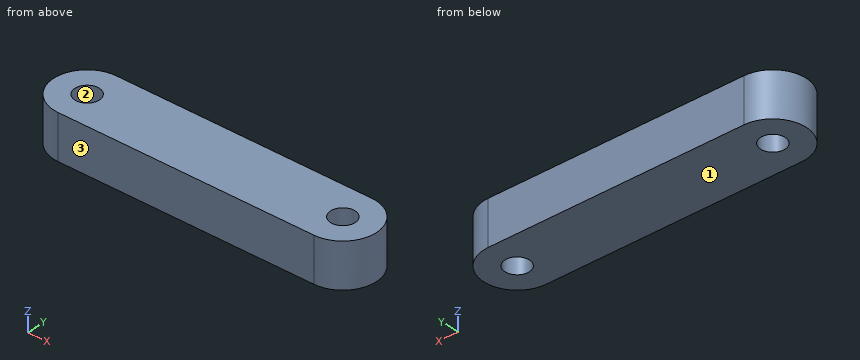
Autodesk Inventor part; units mm, degrees
ref_plane "YZ Plane" through (0, 0, 0) normal (1, 0, 0) x (0, 1, 0)
ref_plane "XZ Plane" through (0, 0, 0) normal (0, 1, 0) x (-1, 0, 0)
ref_plane "XY Plane" through (0, 0, 0) normal (0, 0, 1) x (1, 0, 0)
sketch "Sketch1" plane through (0, 0, 0) normal (0, 0, 1) x (1, 0, 0)
  line L0 (0, 0) -> (36.5125, 0) construction
  line L1 (0, -4.7625) -> (36.5125, -4.7625)
  line L2 (36.5125, 4.7625) -> (0, 4.7625)
  arc A0 (0, 4.7625) -> (0, -4.7625) centre (0, 0) ccw
  arc A1 (36.5125, -4.7625) -> (36.5125, 4.7625) centre (36.5125, 0) ccw
  circle A2 centre (0, 0) radius 1.7526
  circle A3 centre (36.5125, 0) radius 1.7526
  point P0 (18.2563, 0)
  dimension "d0" = 36.5125
  dimension "d1" = 9.525
  dimension "d2" = 3.5052
  dimension "d3" = 3.5052
extrude "Extrusion1" add sketch "Sketch1" along normal blind 6.35
equation "\"d0\" = Rail_Offset"
equation "\"d3\" = d2"
properties part number "Sliders" material "UHMW, White"
For this review, take the finished solid that the model builds, in its own axes (mm). Face numbers are marked on the shaded views. Coordinates: 2 decimals unless noted, no trailing zeros. Write each loop counter-clockwise with the first axis right and the second up, starting at its lowest first coordinate (ties: lowest second). Pieces come first, ordered by that corner, then holes. Notation, with made-up numbers: (42.25, 75.5) -> (82.25, 75.5) arc R12 ccw to (82.25, 97.5) -> close; hole circle Ø4 at (-14.75, -35.75). An arc over 180 degrees is marked (long way). Put each result on its own line as item: value.
Q1. Take a section at A-A, the plane y = 0. Count the separate pieces of the cut face and the enclosed holes in it, then the cut area to 3 significant figures.
From the geometry:
separate pieces: 3
enclosed holes: 0
area: 248 mm2
Q2. Wall thickness on L1, parallel to X at y = -1.5, z = 3.5; L2, parallel to X at y = 0.5, z = 1.25; L3, parallel to Y at x = 0, z = 2: over which ranges is each line inside the solid? List them lowest first.
From the geometry:
L1: x = -4.52 to -0.91, 0.91 to 35.61, 37.42 to 41.03
L2: x = -4.74 to -1.68, 1.68 to 34.83, 38.19 to 41.25
L3: y = -4.76 to -1.75, 1.75 to 4.76
Q3. The part is to be moulded in two halves that separate along Y. For the marked faces 1, 2 and 3, say which applies: +Y half, -Y half, draft (parallel to the pull), parting line (faces both ways), or undercut.
From the geometry:
face 1: draft
face 2: undercut
face 3: -Y half
Q4. Take a section at B-B, the plane z = 5.5. State the section outline as (x, y) points (1 decimal), then the cut area to 3 significant figures.
From the geometry:
outline: (0, -4.8) -> (36.5, -4.8) arc R4.8 ccw to (36.5, 4.8) -> (0, 4.8) arc R4.8 ccw to start; hole circle Ø3.5 at (0, 0); hole circle Ø3.5 at (36.5, 0)
area: 400 mm2
